Verification items for the finished model (mm, model axes). A direction names the side the tool comes from. Give positions to 0.01 mm unless a question says otherwise; leave off trailing zeros. Loops run counter-clockwise (first coordinate to the right, second up) from the corner with the lowest first, then second, coordinate; pieces in that order, holes last. Notation, with made-up numbers: (62.25, -19.5) - (78.25, -19.5) arc R14 ccw to (78.25, 3.5) - close; hole circle Ø9 at (87, 18). An arc over 180 degrees is marked (long way). One line per item, written item: value. Start each with the question number.
1. Sectioned sample at B-B (z = -3.1). Record the cut outline in (x, y).
2. Access from +Z, -Z, +X, -X, +Y, -Y to the whole of each face (thin tool, end or side, straight path). Record for faces 1 (the cylindrical face through (-63, -2, 0)), 2 (the flat face through (43, 0, 0)).
3. Sectioned sample at A-A (x = 29). Record the cut outline in (y, z), plus the area to 3 significant figures.
4. Scan lines: L1, parallel to Y at x = 33, z = -0.1; L2, parallel to Y at x = 33.5, z = 0.65; L3, parallel to X at y = 0.5, z = -2.75. Record each from-to range of solid material in increasing order. Write a range as [from, to].
5. Gauge pin test, flat ends, axial feed: pin 1 (1.1 mm diameter, centred on x = 2, y = -3, fed in from +Z); pin 2 (1 mm diameter, centred on x = -28, z = -1.5, fed in from -Y); pin 3 (2.5 mm diameter, centred on x = -164.5, y = 3, fed in from +Z). Record the tip position at first contact, or that the pin passes through.
from build123d import *

# Parameters (mm, degrees)
SHAFT_DEPTH      = 43
SHAFT_DEPTH_BACK = 167
SKETCH1_R        = 2
SKETCH2_W        = 1.333333334
SKETCH2_H        = 4
SHAFT_M_DEPTH    = 4.5
SKETCH4_W        = 4
SKETCH4_H        = 1.333333334
SHAFT_R_DEPTH    = 4.5
SKETCH6_W        = 1.333333334
SKETCH6_H        = 4
SHAFT_L_DEPTH    = 4.5


with BuildPart() as part:
    # Sketch1 → Shaft (new, two sides: drawn at the far end of the back side and taken through both)
    with BuildSketch(Plane(origin=(0, 0, 0), x_dir=(0, 0, -1), z_dir=(1, 0, 0)).offset(-SHAFT_DEPTH_BACK)):
        Circle(SKETCH1_R)
    extrude(amount=SHAFT_DEPTH + SHAFT_DEPTH_BACK)

    # Sketch2 → Shaft M (add)
    with BuildSketch(Plane.ZY.offset(167)):
        with Locations((0, 2)):
            Rectangle(SKETCH2_W, SKETCH2_H)
    extrude(amount=-SHAFT_M_DEPTH)

    # Sketch4 → Shaft R (add)
    with BuildSketch(Plane(origin=(43, 0, 0), x_dir=(0, 0, -1), z_dir=(1, 0, 0))):
        with Locations((2, 0)):
            Rectangle(SKETCH4_W, SKETCH4_H)
    extrude(amount=-SHAFT_R_DEPTH)

    # Sketch6 → Shaft L (add)
    with BuildSketch(Plane(origin=(0, 0, 0), x_dir=(0, 0, -1), z_dir=(1, 0, 0))):
        with Locations((0, -2)):
            Rectangle(SKETCH6_W, SKETCH6_H)
    extrude(amount=SHAFT_L_DEPTH)


solid = part.part
Results are:
1. outline: (38.5, -0.67) - (43, -0.67) - (43, 0.67) - (38.5, 0.67) - close
2. face 1: none
2. face 2: +Z, -Z, +X, +Y, -Y
3. outline: circle Ø4 at (0, 0)
3. area: 12.6 mm^2
4. L1: y = [-2, 2]
4. L2: y = [-1.89, 1.89]
4. L3: x = [38.5, 43]
5. pin 1: stops at z = 0.67
5. pin 2: stops at y = -1.73
5. pin 3: stops at z = 0.97
